Source: CAD feature listing. Evaluate the final solid. Frame: model axes, mm. A direction names the side the tool comes from. Coordinates: 2 decimals unless noted, no trailing zeros. Loops run counter-clockwise (first coordinate to the right, second up) from the corner with the lowest first, then second, coordinate; pieces in that order, holes last. Notation, with made-up numbers: (61.25, 18) - (72.25, 18) arc R23 cw to (72.25, 35) - close; hole circle Ø11 at (66, -27.5). An arc over 180 degrees is marked (long way). Use CSV: the item, a comma, the result in double quotes. Start each with the question number.
```python
from build123d import *

# Parameters (mm, degrees)
SKETCH1_R           = 45
SKETCH1_R_2         = 1.5
SKETCH1_R_3         = 35
BOSS_EXTRUDE1_DEPTH = 8
CUT_EXTRUDE1_DEPTH  = 2
CUT_EXTRUDE2_START  = -2
CUT_EXTRUDE2_DEPTH  = 2
SKETCH4_R           = 6
CUT_EXTRUDE3_DEPTH  = 10


with BuildPart() as part:
    # Sketch1 → Boss-Extrude1 (new body)
    with BuildSketch(Plane(origin=(0, 0, 0), x_dir=(1, 0, 0), z_dir=(0, 1, 0))):
        with Locations(Location((0, 0, 0), (0, 0, 270))):
            Circle(SKETCH1_R)
        with Locations(Location((0, 40, 0), (0, 0, 270))):
            Circle(SKETCH1_R_2, mode=Mode.SUBTRACT)
        with Locations(Location((40, 0, 0), (0, 0, 270))):
            Circle(SKETCH1_R_2, mode=Mode.SUBTRACT)
        with Locations(Location((0, -40, 0), (0, 0, 270))):
            Circle(SKETCH1_R_2, mode=Mode.SUBTRACT)
        with Locations(Location((-40, 0, 0), (0, 0, 270))):
            Circle(SKETCH1_R_2, mode=Mode.SUBTRACT)
        with Locations(Location((0, 0, 0), (0, 0, 270))):
            Circle(SKETCH1_R_3, mode=Mode.SUBTRACT)
        with Locations(Location((6.945927107, 39.39231012, 0), (0, 0, 270))):
            Circle(SKETCH1_R_2, mode=Mode.SUBTRACT)
        with Locations(Location((-6.945927107, 39.39231012, 0), (0, 0, 270))):
            Circle(SKETCH1_R_2, mode=Mode.SUBTRACT)
        with Locations(Location((39.39231012, 6.945927107, 0), (0, 0, 270))):
            Circle(SKETCH1_R_2, mode=Mode.SUBTRACT)
        with Locations(Location((39.39231012, -6.945927107, 0), (0, 0, 270))):
            Circle(SKETCH1_R_2, mode=Mode.SUBTRACT)
        with Locations(Location((6.945927107, -39.39231012, 0), (0, 0, 270))):
            Circle(SKETCH1_R_2, mode=Mode.SUBTRACT)
        with Locations(Location((-6.945927107, -39.39231012, 0), (0, 0, 270))):
            Circle(SKETCH1_R_2, mode=Mode.SUBTRACT)
        with Locations(Location((-39.39231012, -6.945927107, 0), (0, 0, 270))):
            Circle(SKETCH1_R_2, mode=Mode.SUBTRACT)
        with Locations(Location((-39.39231012, 6.945927107, 0), (0, 0, 270))):
            Circle(SKETCH1_R_2, mode=Mode.SUBTRACT)
    extrude(amount=BOSS_EXTRUDE1_DEPTH)

    # Sketch2 → Cut-Extrude1 (cut)
    with BuildSketch(Plane(origin=(0, 8, 0), x_dir=(1, 0, 0), z_dir=(0, 1, 0))):
        with BuildLine():
            ThreePointArc((10.427551367, 36.541294072), (26.870057685, 26.870057685), (36.541294072, 10.427551367))
            ThreePointArc((36.541294072, 10.427551367), (38.388510428, 11.332541539), (40.445469638, 11.320953396))
            ThreePointArc((40.445469638, 11.320953396), (29.69848481, 29.69848481), (11.320953396, 40.445469638))
            ThreePointArc((11.320953396, 40.445469638), (11.332541539, 38.388510428), (10.427551367, 36.541294072))
        make_face()
        with BuildLine():
            ThreePointArc((40.445469638, -11.320953396), (38.388510428, -11.332541539), (36.541294072, -10.427551367))
            ThreePointArc((36.541294072, -10.427551367), (26.870057685, -26.870057685), (10.427551367, -36.541294072))
            ThreePointArc((10.427551367, -36.541294072), (11.332541539, -38.388510428), (11.320953396, -40.445469638))
            ThreePointArc((11.320953396, -40.445469638), (29.69848481, -29.69848481), (40.445469638, -11.320953396))
        make_face()
        with BuildLine():
            ThreePointArc((-36.541294072, 10.427551367), (-26.870057685, 26.870057685), (-10.427551367, 36.541294072))
            ThreePointArc((-10.427551367, 36.541294072), (-11.332541539, 38.388510428), (-11.320953396, 40.445469638))
            ThreePointArc((-11.320953396, 40.445469638), (-29.69848481, 29.69848481), (-40.445469638, 11.320953396))
            ThreePointArc((-40.445469638, 11.320953396), (-38.388510428, 11.332541539), (-36.541294072, 10.427551367))
        make_face()
        with BuildLine():
            ThreePointArc((-11.320953396, -40.445469638), (-11.332541539, -38.388510428), (-10.427551367, -36.541294072))
            ThreePointArc((-10.427551367, -36.541294072), (-26.870057685, -26.870057685), (-36.541294072, -10.427551367))
            ThreePointArc((-36.541294072, -10.427551367), (-38.388510428, -11.332541539), (-40.445469638, -11.320953396))
            ThreePointArc((-40.445469638, -11.320953396), (-29.69848481, -29.69848481), (-11.320953396, -40.445469638))
        make_face()
    extrude(amount=-CUT_EXTRUDE1_DEPTH, mode=Mode.SUBTRACT)

    # Sketch3 → Cut-Extrude2 (cut)
    with BuildSketch(Plane.XZ.offset(CUT_EXTRUDE2_START)):
        with BuildLine():
            ThreePointArc((10.427551367, 36.541294072), (26.870057685, 26.870057685), (36.541294072, 10.427551367))
            ThreePointArc((36.541294072, 10.427551367), (38.388510428, 11.332541539), (40.445469638, 11.320953396))
            ThreePointArc((40.445469638, 11.320953396), (29.69848481, 29.69848481), (11.320953396, 40.445469638))
            ThreePointArc((11.320953396, 40.445469638), (11.332541539, 38.388510428), (10.427551367, 36.541294072))
        make_face()
        with BuildLine():
            ThreePointArc((40.445469638, -11.320953396), (38.388510428, -11.332541539), (36.541294072, -10.427551367))
            ThreePointArc((36.541294072, -10.427551367), (26.870057685, -26.870057685), (10.427551367, -36.541294072))
            ThreePointArc((10.427551367, -36.541294072), (11.332541539, -38.388510428), (11.320953396, -40.445469638))
            ThreePointArc((11.320953396, -40.445469638), (29.69848481, -29.69848481), (40.445469638, -11.320953396))
        make_face()
        with BuildLine():
            ThreePointArc((-36.541294072, 10.427551367), (-26.870057685, 26.870057685), (-10.427551367, 36.541294072))
            ThreePointArc((-10.427551367, 36.541294072), (-11.332541539, 38.388510428), (-11.320953396, 40.445469638))
            ThreePointArc((-11.320953396, 40.445469638), (-29.69848481, 29.69848481), (-40.445469638, 11.320953396))
            ThreePointArc((-40.445469638, 11.320953396), (-38.388510428, 11.332541539), (-36.541294072, 10.427551367))
        make_face()
        with BuildLine():
            ThreePointArc((-11.320953396, -40.445469638), (-11.332541539, -38.388510428), (-10.427551367, -36.541294072))
            ThreePointArc((-10.427551367, -36.541294072), (-26.870057685, -26.870057685), (-36.541294072, -10.427551367))
            ThreePointArc((-36.541294072, -10.427551367), (-38.388510428, -11.332541539), (-40.445469638, -11.320953396))
            ThreePointArc((-40.445469638, -11.320953396), (-29.69848481, -29.69848481), (-11.320953396, -40.445469638))
        make_face()
    extrude(amount=CUT_EXTRUDE2_DEPTH, mode=Mode.SUBTRACT)

    # Sketch4 → Cut-Extrude3 (cut)
    with BuildSketch(Plane(origin=(0, 0, 0), x_dir=(-1, 0, 0), z_dir=(0, -1, 0))):
        with Locations((0, 50)):
            Circle(SKETCH4_R)
        with Locations((50, 0)):
            Circle(SKETCH4_R)
        with Locations((0, -50)):
            Circle(SKETCH4_R)
        with Locations((-50, 0)):
            Circle(SKETCH4_R)
    extrude(amount=-CUT_EXTRUDE3_DEPTH, mode=Mode.SUBTRACT)


solid = part.part
```
(1) Draft query along Z for faces 3 (the flat face through (-33, 0, 13)), 4 (the cylindrical face through (27.06, 7.01, 26.68)), 5 (the cylindrical face through (0, 4, -44)). Return one class per face: released by +Z, released by -Z, zero draft, split by the parting line, or undercut.
(2) Section D-D on x = -27. Output: boundary loops of the cut face in (y, z).
(3) Section C-C on z = -29.5. Output: boundary loops of the cut face in (x, y).
(4) Section A-A on z = 0. Output: boundary loops of the cut face in (x, y), plus the area to 3 significant figures.
(5) Ray query, line 1 (X direction, y = 7, z = 0); line 2 (X direction, y = 1.5, z = 13.5); line 3 (Z direction, x = -7, y = 4.5). Return the intervals inside material, ascending. Write a range as [from, to].
(6) Section B-B on x = 0. Output: boundary loops of the cut face in (y, z).
(7) Pin query (flat end, axial travel): pin 1 Ø4 at (y, z) = (6.5, 8.5) entering from +X; pin 2 Ø1.5 at (x, y) = (-32, 6) entering from -Z; pin 3 Ø3 at (y, z) = (1.5, 30) entering from -X. Return the tip coordinate at first contact, or that it passes through.
(8) Reachability of faces 1 (the flat face through (-27, 6, 28)), 2 (the cylindrical face through (-38.942, 3.944, 8.377)) from +Z, -Z, +X, -X, +Y, -Y: full face, straight path, thin tool, end or side. Return the list, or none.
Solution:
1,face 3,"zero draft"
1,face 4,"undercut"
1,face 5,"released by -Z"
2,outline,"(0, -36) - (8, -36) - (8, -32.17) - (6, -32.17) - (6, -26.74) - (8, -26.74) - (8, -22.27) - (0, -22.27) - (0, -26.74) - (2, -26.74) - (2, -32.17) - (0, -32.17) - close; (0, 22.27) - (8, 22.27) - (8, 26.74) - (6, 26.74) - (6, 32.17) - (8, 32.17) - (8, 36) - (0, 36) - (0, 32.17) - (2, 32.17) - (2, 26.74) - (0, 26.74) - close"
3,outline,"(-33.98, 0) - (-29.9, 0) - (-29.9, 2) - (-23.95, 2) - (-23.95, 0) - (-18.83, 0) - (-18.83, 8) - (-23.95, 8) - (-23.95, 6) - (-29.9, 6) - (-29.9, 8) - (-33.98, 8) - close; (18.83, 0) - (23.95, 0) - (23.95, 2) - (29.9, 2) - (29.9, 0) - (33.98, 0) - (33.98, 8) - (29.9, 8) - (29.9, 6) - (23.95, 6) - (23.95, 8) - (18.83, 8) - close"
4,outline,"(-44, 0) - (-41.5, 0) - (-41.5, 8) - (-44, 8) - close; (-38.5, 0) - (-35, 0) - (-35, 8) - (-38.5, 8) - close; (35, 0) - (38.5, 0) - (38.5, 8) - (35, 8) - close; (41.5, 0) - (44, 0) - (44, 8) - (41.5, 8) - close"
4,area,"96.0 mm²"
5,line 1,"x = [-44, -41.5], [-38.5, -35], [35, 38.5], [41.5, 44]"
5,line 2,"x = [-42.93, -39.77], [-35.52, -32.29], [32.29, 35.52], [39.77, 42.93]"
5,line 3,"z = [-44.45, -40.89], [-37.89, -34.29], [34.29, 37.89], [40.89, 44.45]"
6,outline,"(0, -44) - (8, -44) - (8, -41.5) - (0, -41.5) - close; (0, -38.5) - (8, -38.5) - (8, -35) - (0, -35) - close; (0, 35) - (8, 35) - (8, 38.5) - (0, 38.5) - close; (0, 41.5) - (8, 41.5) - (8, 44) - (0, 44) - close"
7,pin 1,"stops at x = 44.53"
7,pin 2,"stops at z = -32.38"
7,pin 3,"stops at x = -34.82"
8,face 1,"+Y"
8,face 2,"+Y, -Y"
